Part print with two shaded views. Sizes in mm from the minimum x, y, z corner. Round coordinates to 2 decimals unless told otherwise and drop trailing zeros. Loops run counter-clockwise (first coordinate to the right, second up) from the corner with the lowest first, then second, coordinate; pieces in that order, holes last. Notation, with made-up numbers: (81.5, 6) -> (112.5, 6) arc R23 cw to (112.5, 41) -> close; hole circle Ø6 at (-18, 83). An arc over 180 degrees is marked (long way). Use a Markdown table: item, result. Add a question column.
Item 1: Cut at C-C, the plane z = 0.7. State how many separate pieces and enclosed holes the cut face has, plus the area to 3 significant figures.
Item 2: Cut at A-A, the plane x = 6.35. List the corners of the cut face in (y, z), plus the area to 3 significant figures.
Item 3: Flat gauge pin, fed straight in: pin 1 (5 mm diameter, centred on x = 6.35, y = 149.225, fed in from +Z). Where does the tip first touch, or does it go through?
Item 4: Probe line 1 (Y direction, x = 6.35, z = 0.7); line 2 (Y direction, x = 47.5, z = 1.2); line 3 (X direction, y = 7.5, z = 0.3). List the from-to ranges inside material, lowest first. Write a range as [from, to].
Item 5: Cut at B-B, the plane y = 134.5. List the corners of the cut face in (x, z).
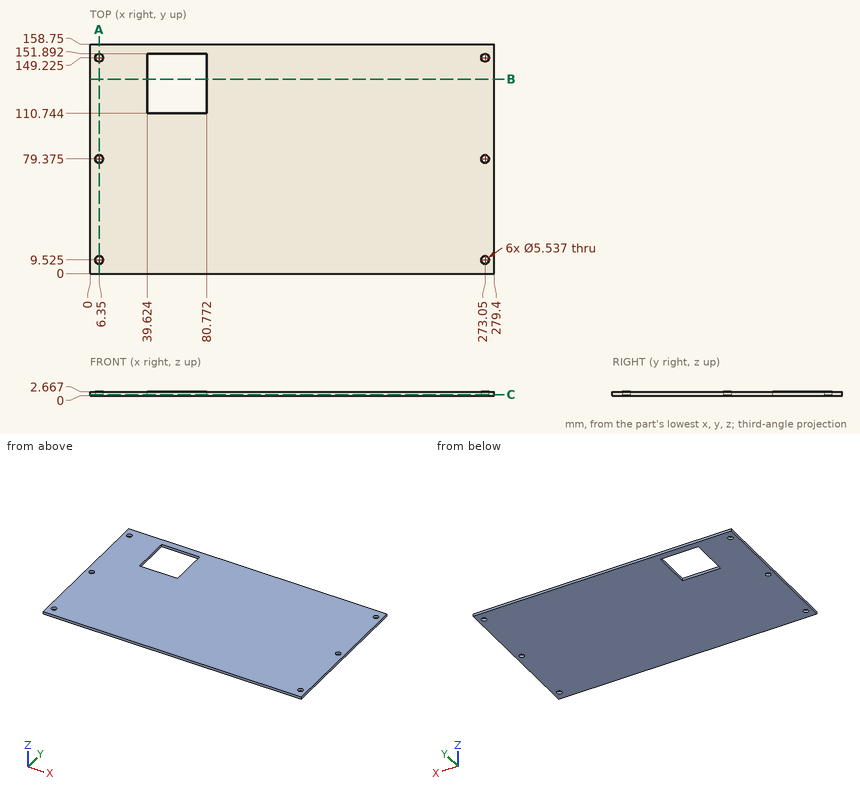
A:
| question | item | result |
|---|---|---|
| 1 | separate pieces | 1 |
| 1 | enclosed holes | 7 |
| 1 | area | 42,500 mm^2 |
| 2 | outline | (0, 0) -> (6.76, 0) -> (6.76, 2.67) -> (0, 2.67) -> close; (12.29, 0) -> (76.61, 0) -> (76.61, 2.67) -> (12.29, 2.67) -> close; (82.14, 0) -> (146.46, 0) -> (146.46, 2.67) -> (82.14, 2.67) -> close; (151.99, 0) -> (158.75, 0) -> (158.75, 2.67) -> (151.99, 2.67) -> close |
| 2 | area | 379 mm^2 |
| 3 | pin 1 | passes through |
| 4 | line 1 | y = [0, 6.76], [12.29, 76.61], [82.14, 146.46], [151.99, 158.75] |
| 4 | line 2 | y = [0, 110.74], [151.89, 158.75] |
| 4 | line 3 | x = [0, 4.46], [8.24, 271.16], [274.94, 279.4] |
| 5 | outline | (0, 0) -> (39.62, 0) -> (39.62, 2.67) -> (0, 2.67) -> close; (80.77, 0) -> (279.4, 0) -> (279.4, 2.67) -> (80.77, 2.67) -> close |
